The listing builds one solid part. Answer for the finished solid, in the listing's coordinates (mm). A direction names the side the tool comes from. Coordinates: 2 decimals unless noted, no trailing zeros. Order: outer loops, then holes, each group sorted by start corner. A loop starts at its lowest first (then second) coordinate and runs counter-clockwise, first axis right, second up.
from build123d import *

# Parameters (mm, degrees)
BOSS_EXTRUDE2_DEPTH = 1


with BuildPart() as part:
    # Sketch1 → Boss-Extrude2 (new body)
    with BuildSketch(Plane.XY):
        with BuildLine():
            Line((-4, 8), (4, 8))
            ThreePointArc((4, 8), (6.828427125, 6.828427125), (8, 4))
            Line((8, 4), (8, -8))
            Line((8, -8), (-8, -8))
            Line((-8, -8), (-8, 4))
            ThreePointArc((-8, 4), (-6.828427125, 6.828427125), (-4, 8))
        make_face()
        with BuildLine():
            Line((-4, 6), (4, 6))
            ThreePointArc((4, 6), (5.414213562, 5.414213562), (6, 4))
            Line((6, 4), (6, -6))
            Line((6, -6), (-6, -6))
            Line((-6, -6), (-6, 4))
            ThreePointArc((-6, 4), (-5.414213562, 5.414213562), (-4, 6))
        make_face(mode=Mode.SUBTRACT)
    extrude(amount=BOSS_EXTRUDE2_DEPTH)


solid = part.part
1) Determine the mould class of faces 3 (the face through (-0.1, 8, 0.5)), 4 (the face through (-8, -2.1, 0.5)), 5 (the face through (-6, -1.1, 0.5)), 6 (the face through (0.1, -8, 0.5)) for opening direction Y: released by +Y, released by -Y, zero draft, split by the parting line, or undercut.
2) Section A-A (y = -3.75) is taken. Give the vertices of the cut face in (x, z), then the cut area to 3 significant figures.
3) Each of these flat-tipped pins is pushed along its axis until it touches: P1, Ø5, axis at x = 3, y = 5, coming from the +Z side; P2, Ø3, axis at x = 0, y = 3, coming from the +Z side. Where does it stop, or does it pass through?
4) A tool of negligible diameter and unlimited length cuts with its end or side. For faces 1 (the face through (0, -7, 1)), 2 (the face through (6, -0.9, 0.5)), from which of +Z, -Z, +X, -X, +Y, -Y can it reach the whole face along a straight path? Write none if from no direction.
5) Section C-C (z = 0.6) is taken. Give the vertices of the cut face in (x, y), then the cut area to 3 significant figures.
6) Consider L1, parallel to X at y = 3, z = 0.15; L2, parallel to Y at x = 5.5, z = 0.5. Determine where each line is inside the solid, lowest interval first.
Filled sheet:
1. face 3: released by +Y
1. face 4: zero draft
1. face 5: undercut
1. face 6: released by -Y
2. outline: (-8, 0) - (-6, 0) - (-6, 1) - (-8, 1) - close; (6, 0) - (8, 0) - (8, 1) - (6, 1) - close
2. area: 4.00 mm2
3. P1: stops at z = 1
3. P2: passes through
4. face 1: +Z, +X, -X, +Y, -Y
4. face 2: +Z, -Z
5. outline: (-8, -8) - (8, -8) - (8, 4) arc R4 ccw to (4, 8) - (-4, 8) arc R4 ccw to (-8, 4) - close; hole (-6, -6) - (6, -6) - (6, 4) arc R2 ccw to (4, 6) - (-4, 6) arc R2 ccw to (-6, 4) - close
5. area: 107 mm2
6. L1: x = -8 to -6, 6 to 8
6. L2: y = -8 to -6, 5.32 to 7.71
